The listing builds one solid part. Answer for the finished solid, in the listing's coordinates (mm). A direction names the side the tool comes from. Give positions to 0.01 mm unless a question says otherwise; leave off trailing zeros. Write each loop counter-clockwise with the first axis right and the second up, starting at its lowest first coordinate (ties: lowest second). Pieces come first, ordered by that corner, then holes. Notation, with made-up numbers: (20, 34.5) -> (25, 34.5) arc R14 cw to (25, 54.5) -> close; hole circle Ø5 at (70.5, 87). An arc over 180 degrees is marked (long way). Write each question's results on one line, items separated by ' | '. Start each with the question number.
from build123d import *

# Parameters (mm, degrees)
BOSS_EXTRUDE1_DEPTH     = 25
CUT_EXTRUDE1_DEPTH      = 25
CUT_EXTRUDE1_DEPTH_BACK = 25
SKETCH3_W               = 12.7
SKETCH3_H               = 4.815210703
SKETCH4_R               = 0.9
CUT_EXTRUDE2_DEPTH      = 25
FILLET1_R               = 0.5
CUT_EXTRUDE3_DEPTH      = 25
CUT_EXTRUDE3_DEPTH_BACK = 25
SKETCH5_R               = 1


with BuildPart() as part:
    # Sketch2 → Boss-Extrude1 (new body)
    with BuildSketch(Plane(origin=(0, 0, 0), x_dir=(0, 0, -1), z_dir=(1, 0, 0))):
        with BuildLine():
            Line((0, -1.8), (-9.11245155, -1.8))
            Line((-9.11245155, -1.8), (-9.11245155, -0.8))
            Line((-9.11245155, -0.8), (-1.61245155, -0.8))
            ThreePointArc((-1.61245155, -0.8), (0.948683298, 1.529705854), (0, -1.8))
        make_face()
    extrude(amount=BOSS_EXTRUDE1_DEPTH)

    # Sketch3 → Cut-Extrude1 (cut, two sides: drawn at the far end of the back side and taken through both)
    with BuildSketch(Plane(origin=(0, 0, 0), x_dir=(1, 0, 0), z_dir=(0, 1, 0)).offset(-CUT_EXTRUDE1_DEPTH_BACK)):
        with Locations((12.5, 0.107605351)):
            Rectangle(SKETCH3_W, SKETCH3_H)
    extrude(amount=CUT_EXTRUDE1_DEPTH + CUT_EXTRUDE1_DEPTH_BACK, mode=Mode.SUBTRACT)

    # Sketch4 → Cut-Extrude2 (cut)
    with BuildSketch(Plane(origin=(25, 0, 0), x_dir=(0, 0, -1), z_dir=(1, 0, 0))):
        Circle(SKETCH4_R)
    extrude(amount=-CUT_EXTRUDE2_DEPTH, mode=Mode.SUBTRACT)

    # Fillet1
    fillet1_edges = [part.edges().sort_by_distance(p)[0] for p in [
        (25, -1.3, 9.11245155),
        (0, -1.3, 9.11245155),
    ]]
    fillet(fillet1_edges, radius=FILLET1_R)

    # Sketch5 → Cut-Extrude3 (cut, two sides: drawn at the far end of the back side and taken through both)
    with BuildSketch(Plane(origin=(0, 0, 0), x_dir=(1, 0, 0), z_dir=(0, 1, 0)).offset(-CUT_EXTRUDE3_DEPTH_BACK)):
        with Locations(Location((5, -5.525991782, 0), (0, 0, 90))):
            Circle(SKETCH5_R)
        with Locations(Location((20, -5.525991782, 0), (0, 0, 90))):
            Circle(SKETCH5_R)
    extrude(amount=CUT_EXTRUDE3_DEPTH + CUT_EXTRUDE3_DEPTH_BACK, mode=Mode.SUBTRACT)


solid = part.part
1. Consider probe 1 along Z at (x, y) = (19.25, -0.1); probe 2 along X at (y, z) = (-1.15, 1.75); probe 3 along Y at (x, z) = (22.75, 0). Determine where each line is inside the solid, lowest interval first. Write a range as [from, to].
2. Section A-A (x = 5) is taken. Write down the section's boundary in (y, z).
3. A tool of negligible diameter and unlimited length cuts with its end or side. For faces 4 (the cylindrical face through (20.976, -1.307, 5.743)), 5 (the flat face through (6.15, -1, 1)), from which of +Z, -Z, +X, -X, +Y, -Y can it reach the whole face along a straight path? Write none if from no direction.
4. Section D-D (z = 1.25) is taken. Write down the section's boundary in (x, y).
5. Each of these flat-tipped pins is pushed along its axis until it touches: pin 1 Ø1.5 at (x, y) = (17.5, -1) entering from -Z; pin 2 Ø1.5 at (x, z) = (13.5, 7) entering from +Y; pin 3 Ø1.1 at (y, z) = (0, 0) entering from +X; pin 4 Ø2.5 at (x, z) = (5, 5.53) entering from -Y. Where does it stop, or does it pass through?
6. Section B-B (y = 0) is taken. Write down the section's boundary in (x, z).
7. The mould has two halves that part along Z. Classify faces 1 (the flat face through (12, -0.8, 5)), 2 (the flat face through (12, -1, 2.3)), 3 (the cylindrical face through (3.12, 0.27, -0.86)): pulls with the +Z half, pulls with the -Z half, needs draft (parallel to the pull), parting line crosses it, or undercut.
8. Section C-C (y = 1.35) is taken. Write down the section's boundary in (x, z).
Results:
1) probe 1: z = [-1.8, -0.89], [0.89, 1.8] | probe 2: x = [0, 6.15], [18.85, 25] | probe 3: y = [-1.8, -0.9], [0.9, 1.8]
2) outline: (-1.8, 0) arc R1.8 ccw (long way) to (-0.8, 1.61) -> (-0.8, 4.53) -> (-1.8, 4.53) -> close; (-1.8, 6.53) -> (-0.8, 6.53) -> (-0.8, 9.11) -> (-1.8, 9.11) -> close; hole circle Ø1.8 at (0, 0)
3) face 4: +Y, -Y | face 5: -Z, +Y, -Y
4) outline: (0, -1.8) -> (6.15, -1.8) -> (6.15, 1.3) -> (0, 1.3) -> close; (18.85, -1.8) -> (25, -1.8) -> (25, 1.3) -> (18.85, 1.3) -> close
5) pin 1: stops at z = 2.3 | pin 2: stops at y = -0.8 | pin 3: passes through | pin 4: stops at y = -1.8
6) outline: (0, -1.8) -> (6.15, -1.8) -> (6.15, -0.9) -> (0, -0.9) -> close; (0, 0.9) -> (6.15, 0.9) -> (6.15, 1.8) -> (0, 1.8) -> close; (18.85, -1.8) -> (25, -1.8) -> (25, -0.9) -> (18.85, -0.9) -> close; (18.85, 0.9) -> (25, 0.9) -> (25, 1.8) -> (18.85, 1.8) -> close
7) face 1: needs draft | face 2: pulls with the -Z half | face 3: undercut
8) outline: (0, -1.19) -> (6.15, -1.19) -> (6.15, 1.19) -> (0, 1.19) -> close; (18.85, -1.19) -> (25, -1.19) -> (25, 1.19) -> (18.85, 1.19) -> close
